from build123d import *

# Parameters (mm, degrees)
BOSS_EXTRUDE1_DEPTH                               = 10.16
SKETCH2_R                                         = 1.4859
CUT_EXTRUDE2_DEPTH                                = 157.71111347
CUT_EXTRUDE3_REACH                                = 158.711
SKETCH3_R                                         = 1.4224
CSK_FOR_3_FLAT_HEAD_MACHINE_SCREW_100_D           = 2.794
CSK_FOR_3_FLAT_HEAD_MACHINE_SCREW_100_CSINK_D     = 7.7978
CSK_FOR_3_FLAT_HEAD_MACHINE_SCREW_100_CSINK_ANGLE = 82


with BuildPart() as part:
    # Sketch1 → Boss-Extrude1 (new body)
    with BuildSketch(Plane(origin=(0, 0, 0), x_dir=(0, 0, -1), z_dir=(1, 0, 0))):
        with BuildLine():
            Line((-136.560270522, -76.2), (41.239729478, -76.2))
            Line((41.239729478, -76.2), (41.239729478, -66.04))
            Line((41.239729478, -66.04), (-115.357986338, -66.04))
            ThreePointArc((-115.357986338, -66.04), (-120.636166121, -63.220342502), (-121.226894187, -57.265454545))
            ThreePointArc((-121.226894187, -57.265454545), (-93.164110025, -23.021842608), (-50.8, -10.16))
            Line((-50.8, -10.16), (0, -10.16))
            Line((0, -10.16), (0, 0))
            Line((0, 0), (-50.8, 0))
            ThreePointArc((-50.8, 0), (-108.161276136, -21.802013662), (-136.560270522, -76.2))
        make_face()
    extrude(amount=BOSS_EXTRUDE1_DEPTH)

    # Sketch2 → Cut-Extrude2 (cut, through all)
    with BuildSketch(Plane(origin=(10.16, 0, 0), x_dir=(0, 0, -1), z_dir=(1, 0, 0))):
        with Locations((-7.62, -5.08)):
            Circle(SKETCH2_R)
    extrude(amount=-CUT_EXTRUDE2_DEPTH, mode=Mode.SUBTRACT)

    # Sketch3 → Cut-Extrude3 (cut, up to next)
    with BuildSketch(Plane.XZ.offset(76.2), mode=Mode.PRIVATE) as cut_extrude3_sk1:
        with Locations(Location((3.81, 116.240270522, 0), (0, 0, 270))):
            Circle(SKETCH3_R)
    cut_extrude3_tool1 = extrude(cut_extrude3_sk1.sketch, amount=-CUT_EXTRUDE3_REACH, mode=Mode.PRIVATE) & part.part
    # Sketch3 → Cut-Extrude3 (cut, up to next)
    with BuildSketch(Plane.XZ.offset(76.2), mode=Mode.PRIVATE) as cut_extrude3_sk2:
        with Locations(Location((3.81, 65.440270522, 0), (0, 0, 270))):
            Circle(SKETCH3_R)
    cut_extrude3_tool2 = extrude(cut_extrude3_sk2.sketch, amount=-CUT_EXTRUDE3_REACH, mode=Mode.PRIVATE) & part.part
    add(cut_extrude3_tool1.solids().sort_by_distance((3.81, -76.2, 116.240271))[0], mode=Mode.SUBTRACT)
    add(cut_extrude3_tool2.solids().sort_by_distance((3.81, -76.2, 65.440271))[0], mode=Mode.SUBTRACT)

    # CSK for #3 Flat Head Machine Screw (100)1 (through all)
    with Locations(Plane(origin=(10.16, 0, 0), x_dir=(0, 0, -1), z_dir=(1, 0, 0))):
        with Locations((-7.62, -5.08)):
            csk_for_3_flat_head_machine_screw_100 = CounterSinkHole(CSK_FOR_3_FLAT_HEAD_MACHINE_SCREW_100_D / 2, CSK_FOR_3_FLAT_HEAD_MACHINE_SCREW_100_CSINK_D / 2, counter_sink_angle=CSK_FOR_3_FLAT_HEAD_MACHINE_SCREW_100_CSINK_ANGLE)

    # Mirror1: CSK for #3 Flat Head Machine Screw (100)1 across plane
    add(csk_for_3_flat_head_machine_screw_100.mirror(Plane(origin=(0, 0, 25.4), x_dir=(1, 0, 0), z_dir=(0, 0, -1))), mode=Mode.SUBTRACT)


solid = part.part
The listing builds one solid part. Answer for the finished solid, in the listing's coordinates (mm). A direction names the side the tool comes from. Round coordinates to 2 decimals unless told otherwise and drop trailing zeros. Write each loop counter-clockwise with the first axis right and the second up, starting at its lowest first coordinate (ties: lowest second). Pieces come first, ordered by that corner, then holes. Notation, with made-up numbers: M 19.5,65 L 63.5,65 A30 ccw 63.5,94 Z; hole C 13.5,29.5 d5. An arc over 180 degrees is marked long. Write each question's results on one line, items separated by ' | '. Start each with the question number.
(1) The part is cut by section B-B, the plane z = -25. Write down the section's boundary in (x, y), and give its area (3 significant figures).
(2) Determine the mould class of faces 3 (the flat face through (5, -66.04, 36)), 4 (the flat face through (5, -5, 0)), 5 (the flat face through (5, 0, 25)) for opening direction Y: +Y half, -Y half, draft (parallel to the pull), parting line (faces both ways), or undercut.
(3) The part is cut by section A-A, the plane z = 21. Write down the section's boundary in (x, y), and give its area (3 significant figures).
(4) Find the intervals of material crossed by line 1 (Y direction, x = 3.5, z = 43.18); line 2 (Y direction, x = 5.5, z = 11); line 3 (Y direction, x = 3, z = 7.62), in increasing order.
(5) For faces 1 (the cylindrical face through (5.009, -23.374, 93.685)), 2 (the cylindrical face through (3.74, -5.98, 8.8)), determine the directions among +Z, -Z, +X, -X, +Y, -Y from which every point of the face is accessible in a straight line to the end or side of a thin tool.
(6) Each of these flat-tipped pins is pushed along its axis until it touches: P1, Ø1.7, axis at x = 3.81, z = 65.44, coming from the +Y side; P2, Ø2.5, axis at y = -5.08, z = 7.62, coming from the -X side; P3, Ø1.5, axis at x = 8.5, y = -56, coming from the +Z side; P4, Ø3, axis at y = -5.08, z = 43.18, coming from the +X side. Where does it stop, or does it pass through?
(7) The part is cut by section C-C, the plane y = -43. Write down the section's boundary in (x, z).
(8) The part is cut by section D-D, the plane z = 107. Write down the section's boundary in (x, y).
Worked answers:
1) outline: M 0,-76.2 L 10.16,-76.2 L 10.16,-66.04 L 0,-66.04 Z | area: 103 mm²
2) face 3: undercut | face 4: draft | face 5: +Y half
3) outline: M 0,-76.2 L 10.16,-76.2 L 10.16,-66.04 L 0,-66.04 Z; M 0,-10.16 L 10.16,-10.16 L 10.16,0 L 0,0 Z | area: 206 mm²
4) line 1: y = -76.2 to -66.04, -10.16 to -6.48, -3.68 to 0 | line 2: y = -76.2 to -66.04, -10.16 to 0 | line 3: y = -76.2 to -66.04, -10.16 to -6.57, -3.59 to 0
5) face 1: -Z, +X, -X | face 2: +X, -X
6) P1: stops at y = -1.11 | P2: passes through | P3: stops at z = 131.93 | P4: stops at x = 7.4
7) outline: M 0,113.46 L 10.16,113.46 L 10.16,125.49 L 0,125.49 Z
8) outline: M 0,-76.2 L 10.16,-76.2 L 10.16,-66.04 L 0,-66.04 Z; M 0,-34.9 L 10.16,-34.9 L 10.16,-20.79 L 0,-20.79 Z
